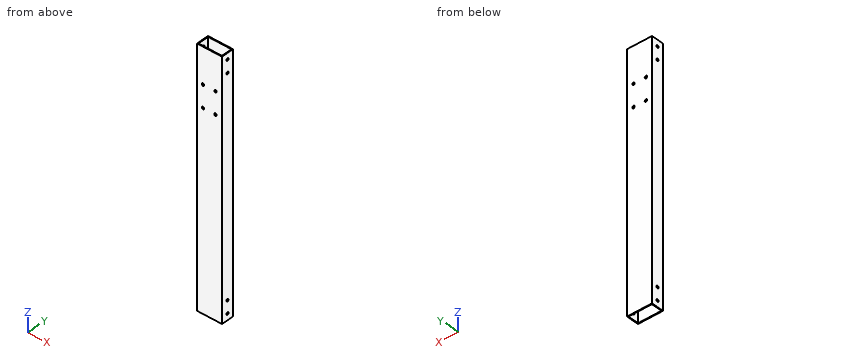
from build123d import *

# Parameters (mm, degrees)
BOSS_EXTRUDE1_DEPTH      = 254.000001
BOSS_EXTRUDE1_DEPTH_BACK = 254.000001
SKETCH3_W                = 50.8
SKETCH3_H                = 25.4
SKETCH3_W_2              = 47.625
SKETCH3_H_2              = 22.225
F_10_CLEARANCE_HOLE1_D   = 4.9784
F_10_CLEARANCE_HOLE2_D   = 4.9784


with BuildPart() as part:
    # Sketch3 → Boss-Extrude1 (new, two sides: drawn at the far end of the back side and taken through both)
    with BuildSketch(Plane.XY.offset(-BOSS_EXTRUDE1_DEPTH_BACK)):
        Rectangle(SKETCH3_W, SKETCH3_H)
        Rectangle(SKETCH3_W_2, SKETCH3_H_2, mode=Mode.SUBTRACT)
    extrude(amount=BOSS_EXTRUDE1_DEPTH + BOSS_EXTRUDE1_DEPTH_BACK)

    # #10 Clearance Hole1 (through all)
    with Locations(Plane(origin=(25.4, 0, 0), x_dir=(0, 0, -1), z_dir=(1, 0, 0))):
        with Locations((-241.300000508, 0), (-215.900000508, 0), (215.899999492, 0), (241.299999492, 0)):
            Hole(F_10_CLEARANCE_HOLE1_D / 2)

    # #10 Clearance Hole2 (through all)
    with Locations(Plane(origin=(0, 12.7, 0), x_dir=(1, 0, 0), z_dir=(0, 1, 0))):
        with Locations((12.19200009, -137.396900508), (-13.20799991, -137.396900508), (-13.20799991, -181.846900508), (12.19200009, -181.846900508)):
            Hole(F_10_CLEARANCE_HOLE2_D / 2)


solid = part.part
Geometry: final body of the model. Coordinates: model frame, mm. Coordinates: 2 decimals unless noted, no trailing zeros. Order: outer loops, then holes, each group sorted by start corner. A loop starts at its lowest first (then second) coordinate and runs counter-clockwise, first axis right, second up. Notation, with made-up numbers: M 9.25,31 L 29.25,31 A15 ccw 29.25,42 Z; hole C -16,77.5 d11. An arc over 180 degrees is marked long. One line per question, with ' | ' between items. Start each with the question number.
Item 1: Cut plane A-A, the plane z = -47. Return the cut outline in (x, y).
Item 2: Cut plane B-B, the plane x = 19. Return the cut outline in (y, z).
Item 3: Ray query, probe 1 along Y at (x, z) = (23, 4.5); probe 2 along X at (y, z) = (-1.5, -85.5); probe 3 along Y at (x, z) = (25, -241.3). Return the intervals inside material, ascending. Write a range as [from, to].
A:
1) outline: M -25.4,-12.7 L 25.4,-12.7 L 25.4,12.7 L -25.4,12.7 Z; hole M -23.81,-11.11 L 23.81,-11.11 L 23.81,11.11 L -23.81,11.11 Z
2) outline: M -12.7,-254 L -11.11,-254 L -11.11,254 L -12.7,254 Z; M 11.11,-254 L 12.7,-254 L 12.7,254 L 11.11,254 Z
3) probe 1: y = [-12.7, -11.11], [11.11, 12.7] | probe 2: x = [-25.4, -23.81], [23.81, 25.4] | probe 3: y = [-12.7, -2.49], [2.49, 12.7]
